```python
from build123d import *

# Parameters (mm, degrees)
SKETCH2_W           = 64.4
SKETCH2_H           = 55.4
SKETCH2_R           = 1.7
BOSS_EXTRUDE1_DEPTH = 5
FILLET1_R           = 5
SKETCH3_R           = 1.7
BOSS_EXTRUDE2_DEPTH = 7


with BuildPart() as part:
    # Sketch2 → Boss-Extrude1 (new body)
    with BuildSketch(Plane(origin=(0, 0, 0), x_dir=(1, 0, 0), z_dir=(0, 1, 0))):
        Rectangle(SKETCH2_W, SKETCH2_H)
        with Locations((-29, 24.5)):
            Circle(SKETCH2_R, mode=Mode.SUBTRACT)
        with Locations((29, 24.5)):
            Circle(SKETCH2_R, mode=Mode.SUBTRACT)
        with Locations((29, -24.5)):
            Circle(SKETCH2_R, mode=Mode.SUBTRACT)
        with Locations((-29, -24.5)):
            Circle(SKETCH2_R, mode=Mode.SUBTRACT)
        Polygon((-26.5, -18.750756585), (-26.5, 18.750756585), (-3.913861386, 0), align=None, mode=Mode.SUBTRACT)
        Polygon((26.5, -18.750756585), (26.5, 18.750756585), (3.913861386, 0), align=None, mode=Mode.SUBTRACT)
        Polygon((-22.586138614, -22), (0, -3.249243415), (22.586138614, -22), align=None, mode=Mode.SUBTRACT)
        Polygon((-22.586138614, 22), (0, 3.249243415), (22.586138614, 22), align=None, mode=Mode.SUBTRACT)
    extrude(amount=BOSS_EXTRUDE1_DEPTH)

    # Fillet1
    fillet1_edges = [part.edges().sort_by_distance(p)[0] for p in [
        (0, 2.5, 3.249243415),
        (3.913861386, 2.5, 0),
        (-3.913861386, 2.5, 0),
        (0, 2.5, -3.249243415),
    ]]
    fillet(fillet1_edges, radius=FILLET1_R)

    # Sketch3 → Boss-Extrude2 (add)
    with BuildSketch(Plane(origin=(0, 5, 0), x_dir=(1, 0, 0), z_dir=(0, 1, 0))):
        with BuildLine():
            Line((-32.2, -21.3), (-32.2, -27.7))
            Line((-32.2, -27.7), (-25.8, -27.7))
            Line((-25.8, -27.7), (-25.8, -24.5))
            ThreePointArc((-25.8, -24.5), (-26.7372583, -22.2372583), (-29, -21.3))
            Line((-29, -21.3), (-32.2, -21.3))
        make_face()
        with Locations((-29, -24.5)):
            Circle(SKETCH3_R, mode=Mode.SUBTRACT)
        with BuildLine():
            Line((-29, 21.3), (-32.2, 21.3))
            Line((-32.2, 21.3), (-32.2, 27.7))
            Line((-32.2, 27.7), (-25.8, 27.7))
            Line((-25.8, 27.7), (-25.8, 24.5))
            ThreePointArc((-25.8, 24.5), (-26.7372583, 22.2372583), (-29, 21.3))
        make_face()
        with Locations((-29, 24.5)):
            Circle(SKETCH3_R, mode=Mode.SUBTRACT)
        with BuildLine():
            Line((25.8, 24.5), (25.8, 27.7))
            Line((25.8, 27.7), (32.2, 27.7))
            Line((32.2, 27.7), (32.2, 21.3))
            Line((32.2, 21.3), (29, 21.3))
            ThreePointArc((29, 21.3), (26.7372583, 22.2372583), (25.8, 24.5))
        make_face()
        with Locations((29, 24.5)):
            Circle(SKETCH3_R, mode=Mode.SUBTRACT)
        with BuildLine():
            Line((25.8, -24.5), (25.8, -27.7))
            Line((25.8, -27.7), (32.2, -27.7))
            Line((32.2, -27.7), (32.2, -21.3))
            Line((32.2, -21.3), (29, -21.3))
            ThreePointArc((29, -21.3), (26.7372583, -22.2372583), (25.8, -24.5))
        make_face()
        with Locations((29, -24.5)):
            Circle(SKETCH3_R, mode=Mode.SUBTRACT)
    extrude(amount=BOSS_EXTRUDE2_DEPTH)


solid = part.part
```
Model file for the job. Use its own axes, mm. A direction names the side the tool comes from. Round coordinates to 2 decimals unless told otherwise and drop trailing zeros. Write each loop counter-clockwise with the first axis right and the second up, starting at its lowest first coordinate (ties: lowest second). Pieces come first, ordered by that corner, then holes. Notation, with made-up numbers: M 45,-8.5 L 103,-8.5 A12 cw 103,0.5 Z; hole C 53,85.5 d11. An arc over 180 degrees is marked long. Put each result on its own line as item: value.
Item 1: Mould opens along Z. For faces 1 (the flat face through (-25.8, 8, 26)), 2 (the cylindrical face through (27, 8, 22)) say: +Z half, -Z half, draft (parallel to the pull), parting line (faces both ways), or undercut.
Responses:
face 1: draft
face 2: undercut
Item 2: Flat gauge pin, fed straight in: P1, Ø10, axis at x = 9, z = 1, coming from the +Y side. Where does the tip first touch, or does it go through?
Responses:
P1: y = 5
Item 3: Cut at C-C (z = 3). List the corners of the cut face in (x, y), and give its area (3 significant figures).
Responses:
outline: M -32.2,0 L -26.5,0 L -26.5,5 L -32.2,5 Z; M -7.74,0 L 7.74,0 L 7.74,5 L -7.74,5 Z; M 26.5,0 L 32.2,0 L 32.2,5 L 26.5,5 Z
area: 134 mm²
Item 4: Cut at A-A (y = 8). List the corners of the cut face in (x, z).
Responses:
outline: M -32.2,-27.7 L -25.8,-27.7 L -25.8,-24.5 A3.2 ccw -29,-21.3 L -32.2,-21.3 Z; M -32.2,21.3 L -29,21.3 A3.2 ccw -25.8,24.5 L -25.8,27.7 L -32.2,27.7 Z; M 25.8,-27.7 L 32.2,-27.7 L 32.2,-21.3 L 29,-21.3 A3.2 ccw 25.8,-24.5 Z; M 25.8,24.5 A3.2 ccw 29,21.3 L 32.2,21.3 L 32.2,27.7 L 25.8,27.7 Z; hole C -29,-24.5 d3.4; hole C -29,24.5 d3.4; hole C 29,-24.5 d3.4; hole C 29,24.5 d3.4
Item 5: Tool access for faces 3 (the flat face through (-30.4, 12, -26)), 4 (the flat face through (31, 8, -21.3)), 5 (the cylindrical face through (-27, 8, 22)), 6 (the flat face through (12.754, 2.465, -13.838)): list every direction of +Z, -Z, +X, -X, +Y, -Y with a clear straight run to the whole face (end or side of a thin tool).
Responses:
face 3: +Z, -Z, +X, -X, +Y
face 4: +X, -X, +Y
face 5: +Y
face 6: +Y, -Y
Item 6: Probe L1, parallel to Z at x = 29, y = 6.5; L2, parallel to X at y = 8, z = -24.5; L3, parallel to X at y = 3, z = -24.5. List the from-to ranges inside material, lowest first. Write a range as from..to.
Responses:
L1: -27.7..-26.2, -22.8..-21.3, 21.3..22.8, 26.2..27.7
L2: -32.2..-30.7, -27.3..-25.8, 25.8..27.3, 30.7..32.2
L3: -32.2..-30.7, -27.3..27.3, 30.7..32.2
Item 7: Cut at B-B (z = 15.5). List the corners of the cut face in (x, y).
Responses:
outline: M -32.2,0 L -26.5,0 L -26.5,5 L -32.2,5 Z; M -22.58,0 L -14.76,0 L -14.76,5 L -22.58,5 Z; M 14.76,0 L 22.58,0 L 22.58,5 L 14.76,5 Z; M 26.5,0 L 32.2,0 L 32.2,5 L 26.5,5 Z
Item 8: Cut at D-D (x = -5). List the corners of the cut face in (y, z).
Responses:
outline: M 0,-27.7 L 5,-27.7 L 5,-22 L 0,-22 Z; M 0,-7.4 L 5,-7.4 L 5,7.4 L 0,7.4 Z; M 0,22 L 5,22 L 5,27.7 L 0,27.7 Z
